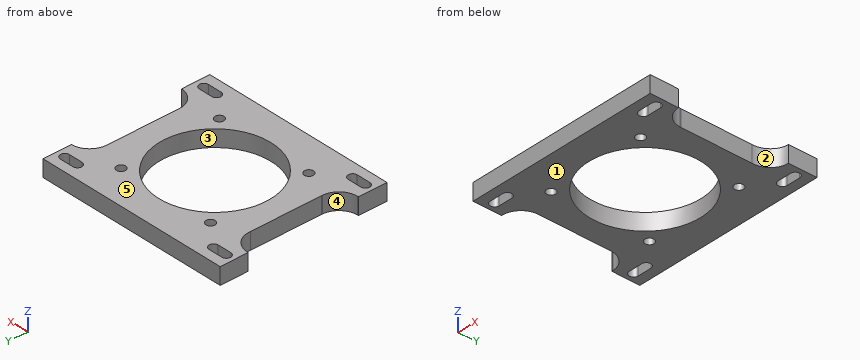
from build123d import *

# Parameters (mm, degrees)
SKETCH1_R           = 40.149801581
SKETCH1_R_2         = 3.249983939
BOSS_EXTRUDE1_DEPTH = 12


with BuildPart() as part:
    # Sketch1 → Boss-Extrude1 (new body)
    with BuildSketch(Plane.XY):
        with BuildLine():
            Line((-68.174111389, 53.990948604), (71.824239973, 54.508639483))
            Line((71.824239973, 54.508639483), (71.899444011, 34.171326758))
            Line((71.899444011, 34.171326758), (71.89945068, 34.169523305))
            ThreePointArc((71.89945068, 34.169523305), (62.293513488, 29.701666637), (58.799882097, 19.700151139))
            Line((58.799882097, 19.700151139), (58.988814164, -31.392458227))
            Line((58.988814164, -31.392458227), (58.990835115, -31.938981122))
            ThreePointArc((58.990835115, -31.938981122), (62.935928372, -41.173957513), (72.156427876, -45.152768721))
            Line((72.156427876, -45.152768721), (72.192770973, -45.15263433))
            Line((72.192770973, -45.15263433), (72.267975011, -65.489947056))
            Line((72.267975011, -65.489947056), (-67.730376351, -66.007637935))
            Line((-67.730376351, -66.007637935), (-67.806147753, -45.51689395))
            Line((-67.806147753, -45.51689395), (-66.849217099, -45.513355378))
            ThreePointArc((-66.849217099, -45.513355378), (-57.65839533, -41.466462132), (-53.781707876, -32.202562082))
            Line((-53.781707876, -32.202562082), (-53.783728828, -31.656039187))
            Line((-53.783728828, -31.656039187), (-53.972660895, 19.436570179))
            ThreePointArc((-53.972660895, 19.436570179), (-57.560711521, 29.434286706), (-67.23952414, 33.810247094))
            Line((-67.23952414, 33.810247094), (-68.099474715, 33.807067138))
            Line((-68.099474715, 33.807067138), (-68.174111389, 53.990948604))
        make_face()
        with Locations((2.046931811, -5.749499226)):
            Circle(SKETCH1_R, mode=Mode.SUBTRACT)
        with Locations((-33.438727493, 29.474686699)):
            Circle(SKETCH1_R_2, mode=Mode.SUBTRACT)
        with Locations((-33.177254114, -41.235158529)):
            Circle(SKETCH1_R_2, mode=Mode.SUBTRACT)
        with Locations((37.532591115, -40.973685151)):
            Circle(SKETCH1_R_2, mode=Mode.SUBTRACT)
        with Locations((37.271117736, 29.736160078)):
            Circle(SKETCH1_R_2, mode=Mode.SUBTRACT)
        with BuildLine():
            Line((65.81073891, -52.110366387), (55.810856699, -52.147344307))
            ThreePointArc((55.810856699, -52.147344307), (52.572912804, -55.40932385), (55.834892347, -58.647267744))
            Line((55.834892347, -58.647267744), (65.834774558, -58.610289825))
            ThreePointArc((65.834774558, -58.610289825), (69.072718453, -55.348310282), (65.81073891, -52.110366387))
        make_face(mode=Mode.SUBTRACT)
        with BuildLine():
            Line((-61.654525972, -59.235157648), (-51.654643761, -59.198179728))
            ThreePointArc((-51.654643761, -59.198179728), (-48.416699866, -55.936200186), (-51.678679409, -52.698256291))
            Line((-51.678679409, -52.698256291), (-61.67856162, -52.735234211))
            ThreePointArc((-61.67856162, -52.735234211), (-64.916505515, -55.997213753), (-61.654525972, -59.235157648))
        make_face(mode=Mode.SUBTRACT)
        with BuildLine():
            Line((55.465113149, 41.351554371), (65.46499536, 41.388532291))
            ThreePointArc((65.46499536, 41.388532291), (68.702939255, 44.650511834), (65.440959712, 47.888455729))
            Line((65.440959712, 47.888455729), (55.441077501, 47.851477809))
            ThreePointArc((55.441077501, 47.851477809), (52.203133606, 44.589498266), (55.465113149, 41.351554371))
        make_face(mode=Mode.SUBTRACT)
        with BuildLine():
            Line((-52.048458607, 47.300565825), (-62.048340818, 47.263587905))
            ThreePointArc((-62.048340818, 47.263587905), (-65.286284713, 44.001608363), (-62.024305171, 40.763664468))
            Line((-62.024305171, 40.763664468), (-52.024422959, 40.800642388))
            ThreePointArc((-52.024422959, 40.800642388), (-48.786479064, 44.06262193), (-52.048458607, 47.300565825))
        make_face(mode=Mode.SUBTRACT)
    extrude(amount=BOSS_EXTRUDE1_DEPTH)


solid = part.part
Design review of the part built by this model. Coordinates are the model's own, in mm. Face numbers are marked on the shaded views. A direction names the side the tool comes from. Round coordinates to 2 decimals unless told otherwise and drop trailing zeros. Loops run counter-clockwise (first coordinate to the right, second up) from the corner with the lowest first, then second, coordinate; pieces in that order, holes last. Notation, with made-up numbers: (72, -31.5) - (130, -31.5) arc R8 cw to (130, -27.5) - close; hole circle Ø4 at (22.5, 3). An arc over 180 degrees is marked (long way). One line per item, written item: value. Start each with the question number.
1) Consider section A-A on y = 5. Give the boundary of the cut face in (x, z), then the cut area to 3 significant figures.
2) Consider section B-B on x = 14.5. Give the boundary of the cut face in (y, z).
3) Consider section C-C on z = 8.5. Give the number of separate pieces and of enclosed holes in the cut face, then the cut area to 3 significant figures.
4) Insertion check: pin 1 Ø10.5 at (x, y) = (-33.44, 29.47) entering from +Z; pin 2 Ø4 at (x, y) = (-33.18, -41.24) entering from -Z; pin 3 Ø2 at (x, z) = (17, 2.5) entering from -Y; pin 4 Ø6 at (x, z) = (39.5, 6) entering from -Y. Each pin has a flat end and moves straight along its axis. Give the tip position at first contact, or say it passes through.
5) For the marked faces 4 and 5, list the 3-axis set-ups (+Z, -Z, +X, -X, +Y, -Y) from which the entire face can be reached by the end or side of a thin tool; tool diameter is ignored.
6) To check wall thickness, follow L1, parallel to Y at x = -35, z = 8; L2, parallel to Y at x = -50, z = 11.5; L3, parallel to X at y = 45, z = 3.25. State the ranges of each line that lie inside material, in increasing order. Write a range as from..to.
7) Draft analysis for pull direction X (two halves, no side actions). For the marked faces 1, 2 and 3, state which applies: +X half, -X half, draft (parallel to the pull), parting line (faces both ways), or undercut.
Reported:
1. outline: (-53.92, 0) - (-36.64, 0) - (-36.64, 12) - (-53.92, 12) - close; (40.73, 0) - (58.85, 0) - (58.85, 12) - (40.73, 12) - close
1. area: 425 mm^2
2. outline: (-65.7, 0) - (-43.92, 0) - (-43.92, 12) - (-65.7, 12) - close; (32.42, 0) - (54.3, 0) - (54.3, 12) - (32.42, 12) - close
3. separate pieces: 1
3. enclosed holes: 9
3. area: 9,210 mm^2
4. pin 1: stops at z = 12
4. pin 2: passes through
4. pin 3: stops at y = -65.7
4. pin 4: stops at y = -65.62
5. face 4: +Z, -Z, -X
5. face 5: +Z, +X, -X, +Y, -Y
6. L1: y = -65.89..-43.93, -38.54..-21.23, 9.73..26.62, 32.33..54.11
6. L2: y = -65.94..-58.74, -53.16..41.52, 46.58..54.06
6. L3: x = -68.14..-65.13, -48.93..52.23, 68.68..71.86
7. face 1: draft
7. face 2: +X half
7. face 3: undercut
